from build123d import *

# Parameters (mm, degrees)
SKETCH1_R           = 2
BOSS_EXTRUDE1_DEPTH = 30
SKETCH2_W           = 24
SKETCH2_H           = 15
CUT_EXTRUDE1_DEPTH  = 43.435404183
SKETCH3_R           = 8.9
SKETCH3_R_2         = 2
CUT_EXTRUDE2_DEPTH  = 3


with BuildPart() as part:
    # Sketch1 → Boss-Extrude1 (new body)
    with BuildSketch(Plane.XY):
        with BuildLine():
            Line((-10, 22.377746272), (10, 22.377746272))
            Line((10, 22.377746272), (10, -13.032253728))
            ThreePointArc((10, -13.032253728), (0, -16.426796317), (-10, -13.032253728))
            Line((-10, -13.032253728), (-10, 22.377746272))
        make_face()
        with Locations((0, -7.032253728)):
            Circle(SKETCH1_R, mode=Mode.SUBTRACT)
        with Locations((6, -7.032253728)):
            Circle(SKETCH1_R, mode=Mode.SUBTRACT)
        with Locations((-6, -7.032253728)):
            Circle(SKETCH1_R, mode=Mode.SUBTRACT)
    extrude(amount=BOSS_EXTRUDE1_DEPTH)

    # Sketch2 → Cut-Extrude1 (cut, through all)
    with BuildSketch(Plane(origin=(10, 0, 0), x_dir=(0, 0, -1), z_dir=(1, 0, 0))):
        with Locations((-15, -8.926796317)):
            Rectangle(SKETCH2_W, SKETCH2_H)
    extrude(amount=-CUT_EXTRUDE1_DEPTH, mode=Mode.SUBTRACT)

    # Sketch3 → Cut-Extrude2 (cut)
    with BuildSketch(Plane.ZY.offset(10)):
        with Locations((15, 10.473203683)):
            Circle(SKETCH3_R)
        with Locations((15, 16.473203683)):
            Circle(SKETCH3_R_2, mode=Mode.SUBTRACT)
        with Locations((15, 4.473203683)):
            Circle(SKETCH3_R_2, mode=Mode.SUBTRACT)
        with Locations((9, 10.473203683)):
            Circle(SKETCH3_R_2, mode=Mode.SUBTRACT)
        with Locations((21, 10.473203683)):
            Circle(SKETCH3_R_2, mode=Mode.SUBTRACT)
    extrude(amount=-CUT_EXTRUDE2_DEPTH, mode=Mode.SUBTRACT)


solid = part.part
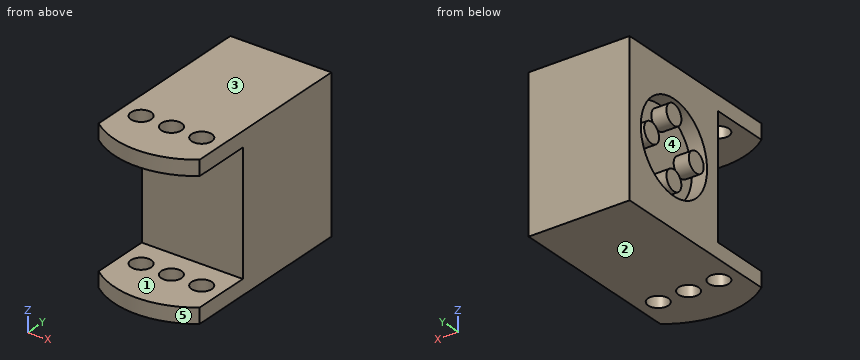
Geometry check sheet. Reference: the model listing, model coordinates, mm. Face numbers are marked on the shaded views. A direction names the side the tool comes from. Coordinates: 2 decimals unless noted, no trailing zeros. Order: outer loops, then holes, each group sorted by start corner. A loop starts at its lowest first (then second) coordinate and runs counter-clockwise, first axis right, second up. Notation, with made-up numbers: (62, 9) - (114, 9) arc R30 ccw to (114, 31) - close; hole circle Ø6 at (85.5, 48.25). An arc over 180 degrees is marked (long way). Answer in a Markdown table with one row per item. Add a question column.
1) Release check for a two-part mould opening along Y. For the marked faces 3, 4 and 5 record: +Y half, -Y half, draft (parallel to the pull), parting line (faces both ways), or undercut.
2) Set-up check for the marked faces 1 and 2: record each of +Z, -Z, +X, -X, +Y, -Y from which the full face is reachable in a straight line by a thin tool's end or side.
3) Cross-section at C-C, the plane x = 0. Record the cut outline in (y, z).
4) Cross-section at A-A, the plane y = -12. Record the cut outline in (x, z), then the cut area to 3 significant figures.
5) Material ranges on line 1 along Z through (x, y) = (-1, -14); line 2 along Y through (x, z) = (0, 28.05); line 3 along Y through (x, z) = (-8.25, 7.75), recorded low to high. Write a range as [from, to].
6) Gauge pin test, flat ends, axial feed: P1, Ø3, axis at x = 8, z = 24.5, coming from the -Y side; P2, Ø2.5, axis at x = -6, y = -7.03, coming from the +Z side. Record the tip position at first contact, or that the pin passes through.
7) Cross-section at B-B, the plane z = 15. Record the cut outline in (x, y), then the cut area to 3 significant figures.
8) Cross-section at D-D, the plane x = -6.25. Record the cut outline in (y, z).
Check result:
| question | item | result |
|---|---|---|
| 1 | face 3 | draft |
| 1 | face 4 | undercut |
| 1 | face 5 | -Y half |
| 2 | face 1 | +X, -X, -Y |
| 2 | face 2 | -Z, +X, -X, +Y, -Y |
| 3 | outline | (-16.43, 0) - (-9.03, 0) - (-9.03, 3) - (-16.43, 3) - close; (-16.43, 27) - (-9.03, 27) - (-9.03, 30) - (-16.43, 30) - close; (-5.03, 0) - (22.38, 0) - (22.38, 30) - (-5.03, 30) - (-5.03, 27) - (-1.43, 27) - (-1.43, 3) - (-5.03, 3) - close |
| 4 | outline | (-10, 0) - (10, 0) - (10, 3) - (-10, 3) - close; (-10, 27) - (10, 27) - (10, 30) - (-10, 30) - close |
| 4 | area | 120 mm² |
| 5 | line 1 | z = [0, 3], [27, 30] |
| 5 | line 2 | y = [-16.43, -9.03], [-5.03, 22.38] |
| 5 | line 3 | y = [-1.43, 5.31], [8.91, 12.03], [15.64, 22.38] |
| 6 | P1 | stops at y = -1.43 |
| 6 | P2 | passes through |
| 7 | outline | (-10, -1.43) - (10, -1.43) - (10, 22.38) - (-10, 22.38) - (-10, 19.37) - (-7, 19.37) - (-7, 18.47) - (-10, 18.47) - (-10, 14.47) - (-7, 14.47) - (-7, 6.47) - (-10, 6.47) - (-10, 2.47) - (-7, 2.47) - (-7, 1.57) - (-10, 1.57) - close |
| 7 | area | 447 mm² |
| 8 | outline | (-15.19, 0) - (-9.02, 0) - (-9.02, 3) - (-15.19, 3) - close; (-15.19, 27) - (-9.02, 27) - (-9.02, 30) - (-15.19, 30) - close; (-5.05, 0) - (22.38, 0) - (22.38, 30) - (-5.05, 30) - (-5.05, 27) - (-1.43, 27) - (-1.43, 3) - (-5.05, 3) - close |
